```python
from build123d import *

# Parameters (mm, degrees)
SKETCH1_R           = 1.45
BOSS_EXTRUDE1_DEPTH = 5


with BuildPart() as part:
    # Sketch1 → Boss-Extrude1 (new body)
    with BuildSketch(Plane.XY.offset(1.9)):
        with BuildLine():
            Line((-13.026395415, 38.955911265), (-0.214852682, -8.857417136))
            ThreePointArc((-0.214852682, -8.857417136), (0.949961883, -10.375433033), (2.847009496, -10.625184089))
            Line((2.847009496, -10.625184089), (5.261824062, -9.978136476))
            Line((5.261824062, -9.978136476), (5.188879797, -9.705904774))
            Line((5.188879797, -9.705904774), (6.08761429, -9.187020173))
            ThreePointArc((6.08761429, -9.187020173), (5.919814799, -7.906537121), (5.481893659, -6.691622066))
            Line((5.481893659, -6.691622066), (5.414116812, -6.552658937))
            ThreePointArc((5.414116812, -6.552658937), (6.01040764, -6.01040764), (6.552658937, -5.414116812))
            Line((6.552658937, -5.414116812), (6.691622066, -5.481893659))
            ThreePointArc((6.691622066, -5.481893659), (7.906537121, -5.919814799), (9.187020173, -6.08761429))
            Line((9.187020173, -6.08761429), (9.86553871, -4.91238571))
            ThreePointArc((9.86553871, -4.91238571), (9.079978562, -3.887354604), (8.093270203, -3.054167872))
            Line((8.093270203, -3.054167872), (7.965092167, -2.967710696))
            ThreePointArc((7.965092167, -2.967710696), (8.210369523, -2.199961883), (8.381827508, -1.41243323))
            Line((8.381827508, -1.41243323), (8.536061531, -1.401648137))
            ThreePointArc((8.536061531, -1.401648137), (9.807169402, -1.173441441), (11, -0.678518537))
            Line((11, -0.678518537), (11, 0.678518537))
            ThreePointArc((11, 0.678518537), (9.807169402, 1.173441441), (8.536061531, 1.401648137))
            Line((8.536061531, 1.401648137), (8.381827508, 1.41243323))
            ThreePointArc((8.381827508, 1.41243323), (8.210369523, 2.199961883), (7.965092167, 2.967710696))
            Line((7.965092167, 2.967710696), (8.093270203, 3.054167872))
            ThreePointArc((8.093270203, 3.054167872), (9.079978562, 3.887354604), (9.86553871, 4.91238571))
            Line((9.86553871, 4.91238571), (9.187020173, 6.08761429))
            ThreePointArc((9.187020173, 6.08761429), (7.906537121, 5.919814799), (6.691622066, 5.481893659))
            Line((6.691622066, 5.481893659), (6.552658937, 5.414116812))
            ThreePointArc((6.552658937, 5.414116812), (6.01040764, 6.01040764), (5.414116812, 6.552658937))
            Line((5.414116812, 6.552658937), (5.481893659, 6.691622066))
            ThreePointArc((5.481893659, 6.691622066), (5.919814799, 7.906537121), (6.08761429, 9.187020173))
            Line((6.08761429, 9.187020173), (4.91238571, 9.86553871))
            ThreePointArc((4.91238571, 9.86553871), (3.887354604, 9.079978562), (3.054167872, 8.093270203))
            Line((3.054167872, 8.093270203), (2.967710696, 7.965092167))
            ThreePointArc((2.967710696, 7.965092167), (2.199961883, 8.210369523), (1.41243323, 8.381827508))
            Line((1.41243323, 8.381827508), (1.401648136, 8.536061531))
            ThreePointArc((1.401648136, 8.536061531), (1.173441441, 9.807169402), (0.678518537, 11))
            Line((0.678518537, 11), (-0.359250666, 11))
            Line((-0.359250666, 11), (-8.196766283, 40.250006491))
            ThreePointArc((-8.196766283, 40.250006491), (-11.258628462, 42.017773444), (-13.026395415, 38.955911265))
        make_face()
        with Locations((-10.611580849, 39.602958878)):
            Circle(SKETCH1_R, mode=Mode.SUBTRACT)
        Circle(SKETCH1_R, mode=Mode.SUBTRACT)
    extrude(amount=-BOSS_EXTRUDE1_DEPTH)


solid = part.part
```
Design review of the part built by this model. Coordinates are the model's own, in mm. A direction names the side the tool comes from. Give positions to 0.01 mm unless a question says otherwise; leave off trailing zeros. Order: outer loops, then holes, each group sorted by start corner. A loop starts at its lowest first (then second) coordinate and runs counter-clockwise, first axis right, second up. Notation, with made-up numbers: M 80.25,-5 L 88.25,-5 A14 cw 88.25,15 Z; hole C 43,66 d5. An arc over 180 degrees is marked long. One line per question, with ' | ' between items. Start each with the question number.
Q1. We need section C-C (x = -4.25). Write out the cut boundary in (y, z).
Q2. Machinability: for faces 1 (the face through (0, 11, -1)), 2 (the face through (7.889, -5.916, -0.565)), 3 (the face through (7.924, 5.924, -0.565)), 4 (the face through (5.916, 7.889, -0.565)), which of the approach directions +Z, -Z, +X, -X, +Y, -Y give a long, thin tool a straight path to every point of the face, cutting with its end or side? Answer none if there is none.
Q3. We need section B-B (y = 0). Write out the cut boundary in (x, z), plus the area to 3 significant figures.
Q4. For L1, parallel to Y at x = 9.25, z = -1.85; L2, parallel to Y at x = 0, z = -0.65; L3, parallel to Y at x = 6.5, z = -1.6, list the stretches that pass through material, from the lowest coordinate up. Write a range as [from, to].
Q5. We need section D-D (z = 0.55). State how many separate pieces and enclosed holes the cut face has, plus the area to 3 significant figures.
Q6. For pin 1 Ø3 at (y, z) = (1, 1) entering from -X; pin 2 Ø2.5 at (x, y) = (0, 0) entering from -Z, all flat-tipped, find the tip position at first contact; note any pin that passes through.
Q7. We need section A-A (x = -11.25). Write out the cut boundary in (y, z), plus the area to 3 significant figures.
Q8. The part is to be moulded in two halves that separate along Y. For faces 5 (the face through (9.09, -3.9, -0.56)), 6 (the face through (-2, 12, -3.1)), 7 (the face through (3.9, 9.09, -0.56)), 8 (the face through (9.52, -5.51, -0.56)), say which applies: +Y half, -Y half, draft (parallel to the pull), parting line (faces both ways), or undercut.
Returned:
1) outline: M 6.2,-3.1 L 25.52,-3.1 L 25.52,1.9 L 6.2,1.9 Z
2) face 1: +Z, -Z, +X, +Y | face 2: +Z, -Z, -Y | face 3: +Z, -Z, +Y | face 4: +Z, -Z, +X
3) outline: M -2.59,-3.1 L -1.45,-3.1 L -1.45,1.9 L -2.59,1.9 Z; M 1.45,-3.1 L 11,-3.1 L 11,1.9 L 1.45,1.9 Z | area: 53.4 mm2
4) L1: [-5.98, -4.07], [-1.31, 1.31], [4.07, 5.98] | L2: [-9.4, -1.45], [1.45, 11] | L3: [-5.48, 5.48]
5) separate pieces: 1 | enclosed holes: 2 | area: 356 mm2
6) pin 1: x = -3.26 | pin 2: through
7) outline: M 32.33,-3.1 L 38.3,-3.1 L 38.3,1.9 L 32.33,1.9 Z; M 40.9,-3.1 L 42.02,-3.1 L 42.02,1.9 L 40.9,1.9 Z | area: 35.4 mm2
8) face 5: undercut | face 6: draft | face 7: +Y half | face 8: -Y half
